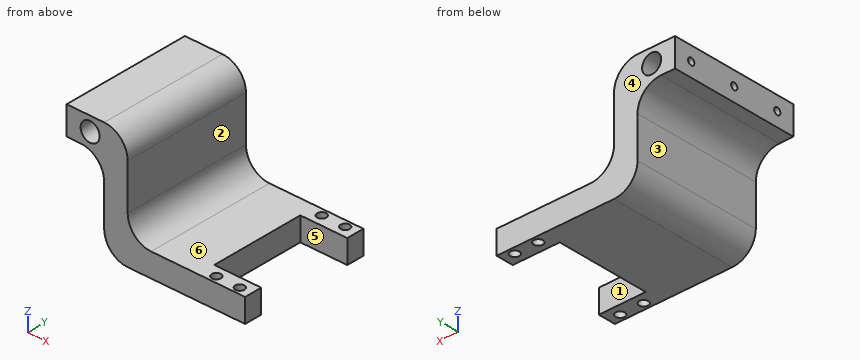
```python
from build123d import *

# Parameters (mm, degrees)
SKETCH1_W           = 20
SKETCH1_H           = 7.5
SKETCH1_R           = 1.95
BOSS_EXTRUDE2_DEPTH = 10
SKETCH3_W           = 49.35
SKETCH3_H           = 55
BOSS_EXTRUDE3_DEPTH = 10
SKETCH4_W           = 16
SKETCH4_H           = 12
SKETCH4_R           = 4.05
BOSS_EXTRUDE4_DEPTH = 55
SKETCH5_R           = 1.45
CUT_EXTRUDE1_DEPTH  = 10
FILLET1_R           = 10


with BuildPart() as part:
    # Sketch1 → Boss-Extrude2 (new body)
    with BuildSketch(Plane.XY):
        Polygon((-10, 27.5), (-40, 27.5), (-40, -27.5), (-10, -27.5), (-10, -20), (-10, 20), align=None)
        with Locations((0, 23.75)):
            Rectangle(SKETCH1_W, SKETCH1_H)
        with Locations((5, 24.5)):
            Circle(SKETCH1_R, mode=Mode.SUBTRACT)
        with Locations((-5, 24.5)):
            Circle(SKETCH1_R, mode=Mode.SUBTRACT)
        with Locations((0, -23.75)):
            Rectangle(SKETCH1_W, SKETCH1_H)
        with Locations((5, -24.5)):
            Circle(SKETCH1_R, mode=Mode.SUBTRACT)
        with Locations((-5, -24.5)):
            Circle(SKETCH1_R, mode=Mode.SUBTRACT)
    extrude(amount=BOSS_EXTRUDE2_DEPTH)

    # Sketch3 → Boss-Extrude3 (add)
    with BuildSketch(Plane.ZY.offset(40)):
        with Locations((24.675, 0)):
            Rectangle(SKETCH3_W, SKETCH3_H)
    extrude(amount=BOSS_EXTRUDE3_DEPTH)

    # Sketch4 → Boss-Extrude4 (add)
    with BuildSketch(Plane.XZ.offset(27.5)):
        with Locations((-58, 43.35)):
            Rectangle(SKETCH4_W, SKETCH4_H)
        with Locations((-56, 43.35)):
            Circle(SKETCH4_R, mode=Mode.SUBTRACT)
    extrude(amount=-BOSS_EXTRUDE4_DEPTH)

    # Sketch5 → Cut-Extrude1 (cut)
    with BuildSketch(Plane.ZY.offset(66)):
        with Locations((43.35, 20)):
            Circle(SKETCH5_R)
        with Locations((43.35, 0)):
            Circle(SKETCH5_R)
        with Locations((43.35, -20)):
            Circle(SKETCH5_R)
    extrude(amount=-CUT_EXTRUDE1_DEPTH, mode=Mode.SUBTRACT)

    # Fillet1
    fillet1_edges = [part.edges().sort_by_distance(p)[0] for p in [
        (-40, 0, 10),
        (-40, 0, 49.35),
        (-50, 0, 0),
        (-50, 0, 37.35),
    ]]
    fillet(fillet1_edges, radius=FILLET1_R)


solid = part.part
```
Geometry: final body of the model. Coordinates: model frame, mm. Face numbers are marked on the shaded views. A direction names the side the tool comes from. Round coordinates to 2 decimals unless told otherwise and drop trailing zeros. Order: outer loops, then holes, each group sorted by start corner. A loop starts at its lowest first (then second) coordinate and runs counter-clockwise, first axis right, second up. Notation, with made-up numbers: (28.5, -13) -> (82.5, -13) arc R25 ccw to (82.5, 15) -> close; hole circle Ø11 at (55.5, 38). An arc over 180 degrees is marked (long way). Use one line per item in the form item = value.
(1) Section A-A on y = -24.5. Return loops of the section in (x, z), and give its area (3 significant figures).
Results list:
outline = (-66, 37.35) -> (-60, 37.35) arc R10 cw to (-50, 27.35) -> (-50, 10) arc R10 ccw to (-40, 0) -> (-6.95, 0) -> (-6.95, 10) -> (-30, 10) arc R10 cw to (-40, 20) -> (-40, 39.35) arc R10 ccw to (-50, 49.35) -> (-66, 49.35) -> close; (-3.05, 0) -> (3.05, 0) -> (3.05, 10) -> (-3.05, 10) -> close; (6.95, 0) -> (10, 0) -> (10, 10) -> (6.95, 10) -> close; hole circle Ø8.1 at (-56, 43.35)
area = 1,060 mm^2
(2) Ray query, probe 1 along Y at (x, z) = (-62, 43.35); probe 2 along Y at (x, z) = (5, 8); probe 3 along Z at (x, y) = (-61, 20). Return the intervals inside material, ascending. Write a range as [from, to].
Results list:
probe_1 = [-27.5, -21.45], [-18.55, -1.45], [1.45, 18.55], [21.45, 27.5]
probe_2 = [-27.5, -26.45], [-22.55, -20], [20, 22.55], [26.45, 27.5]
probe_3 = [37.35, 41.9], [44.8, 49.35]
(3) First-contact query: pin 1 Ø4.5 at (y, z) = (-20, 43.35) entering from -X; pin 2 Ø14 at (y, z) = (-9, 15.5) entering from -X; pin 3 Ø8 at (y, z) = (-8, 20.5) entering from +X; pin 4 Ø2 at (y, z) = (13.5, 13) entering from +X. Flat tips, straight axial feed; report the tip coordinate or a pass-through.
Results list:
pin_1 = -66
pin_2 = -50
pin_3 = -39.37
pin_4 = -36
(4) Section D-D on y = 23.5. Return loops of the section in (x, z), and give its area (3 significant figures).
Results list:
outline = (-66, 37.35) -> (-60, 37.35) arc R10 cw to (-50, 27.35) -> (-50, 10) arc R10 ccw to (-40, 0) -> (-6.67, 0) -> (-6.67, 10) -> (-30, 10) arc R10 cw to (-40, 20) -> (-40, 39.35) arc R10 ccw to (-50, 49.35) -> (-66, 49.35) -> close; (-3.33, 0) -> (3.33, 0) -> (3.33, 10) -> (-3.33, 10) -> close; (6.67, 0) -> (10, 0) -> (10, 10) -> (6.67, 10) -> close; hole circle Ø8.1 at (-56, 43.35)
area = 1,070 mm^2
(5) Draft query along Y for the marked faces 4, 5 and 6. Return one class per face: pulls with the +Y half, pulls with the -Y half, needs draft (parallel to the pull), parting line crosses it, or undercut.
Results list:
face_4 = pulls with the +Y half
face_5 = undercut
face_6 = needs draft
(6) Section B-B on x = 5. Return loops of the section in (y, z).
Results list:
outline = (-27.5, 0) -> (-26.45, 0) -> (-26.45, 10) -> (-27.5, 10) -> close; (-22.55, 0) -> (-20, 0) -> (-20, 10) -> (-22.55, 10) -> close; (20, 0) -> (22.55, 0) -> (22.55, 10) -> (20, 10) -> close; (26.45, 0) -> (27.5, 0) -> (27.5, 10) -> (26.45, 10) -> close
(7) Section C-C on z = 43.35. Return loops of the section in (x, y), and give its area (3 significant figures).
Results list:
outline = (-66, -27.5) -> (-60.05, -27.5) -> (-60.05, -21.45) -> (-66, -21.45) -> close; (-66, -18.55) -> (-60.05, -18.55) -> (-60.05, -1.45) -> (-66, -1.45) -> close; (-66, 1.45) -> (-60.05, 1.45) -> (-60.05, 18.55) -> (-66, 18.55) -> close; (-66, 21.45) -> (-60.05, 21.45) -> (-60.05, 27.5) -> (-66, 27.5) -> close; (-51.95, -27.5) -> (-40.83, -27.5) -> (-40.83, 27.5) -> (-51.95, 27.5) -> close
area = 887 mm^2
(8) Access query for the marked faces 1, 2 and 3. Directions: +Z, -Z, +X, -X, +Y, -Y. A direction counts if a zero-diameter tool reaches every point of the face in a straight line with its end or side. Return the directions, or none.
Results list:
face_1 = +Z, -Z, +X
face_2 = +Z, +X, +Y, -Y
face_3 = -Z, -X, +Y, -Y
